```python
from build123d import *

# Parameters (mm, degrees)
SKETCH_1_W          = 10
SKETCH_1_H          = 10
EXTRUDE_1_DEPTH     = 10
SKETCH_4_R          = 3
CUT_EXTRUDE_2_DEPTH = 11
SKETCH_5_R          = 2.5
CUT_EXTRUDE_3_DEPTH = 11
FILLET_1_R          = 0.5


with BuildPart() as part:
    # 草图1 → 凸台-拉伸1 (new body)
    with BuildSketch(Plane.XY):
        with Locations((5, 5)):
            Rectangle(SKETCH_1_W, SKETCH_1_H)
    extrude(amount=EXTRUDE_1_DEPTH)

    # 草图4 → 切除-拉伸2 (cut, through all)
    with BuildSketch(Plane(origin=(10, 0, 0), x_dir=(0, 0, -1), z_dir=(1, 0, 0))):
        with Locations((-5, 5)):
            Circle(SKETCH_4_R)
    extrude(amount=-CUT_EXTRUDE_2_DEPTH, mode=Mode.SUBTRACT)

    # 草图5 → 切除-拉伸3 (cut, through all)
    with BuildSketch(Plane.XY.offset(10)):
        with Locations((5, 5)):
            Circle(SKETCH_5_R)
    extrude(amount=-CUT_EXTRUDE_3_DEPTH, mode=Mode.SUBTRACT)

    # 圆角1
    fillet_1_edges = [part.edges().sort_by_distance(p)[0] for p in [
        (10, 5, 10),
        (0, 5, 8),
        (10, 5, 8),
        (5, 10, 10),
        (2.5, 5, 0),
        (2.5, 5, 10),
        (0, 5, 10),
        (5, 10, 0),
        (10, 5, 0),
        (5, 0, 0),
        (0, 5, 0),
        (10, 10, 5),
        (10, 0, 5),
        (5, 0, 10),
    ]]
    fillet(fillet_1_edges, radius=FILLET_1_R)


solid = part.part
```
Here's how the part is built. I have some questions about the finished solid (model axes, mm). Coordinates: 2 decimals unless noted, no trailing zeros. Loops run counter-clockwise (first coordinate to the right, second up) from the corner with the lowest first, then second, coordinate; pieces in that order, holes last. Notation, with made-up numbers: (14.5, 32.5) - (60.5, 32.5) arc R20 ccw to (60.5, 71.5) - close; hole circle Ø1 at (8, 42). An arc over 180 degrees is marked (long way). Return JSON: item names as keys, results as strings. Group by question number.
Item 1: We'd pull the mould along Y, two halves only. Please class faces 1 (the face through (5, 10, 5)), 2 (the face through (2, 6, 0)), 3 (the face through (7.385, 5.751, 8.415)): +Y half, -Y half, draft (parallel to the pull), parting line (faces both ways), or undercut.
Item 2: If we section it at D-D on x = 9.25: Write out the boundary of the cut face in (y, z), and give its area (3 significant figures).
Item 3: If we section it at A-A on x = 5: Write out the boundary of the cut face in (y, z).
Item 4: If we section it at C-C on y = 5: Write out the boundary of the cut face in (x, z), and give its area (3 significant figures).
Item 5: I need wall thicknesses on line 1 (Y direction, x = 1.5, z = 7.5); line 2 (Y direction, x = 5, z = 1.65). Which ranges of each line are inside material? Lowest first, please. Write a range as from..to.
Item 6: If we section it at B-B on z = 5: Write out the boundary of the cut face in (x, y).
Calculated:
{
 "1": {"face 1": "+Y half", "face 2": "draft", "face 3": "undercut"},
 "2": {"outline": "(0, 0.5) arc R0.5 ccw to (0.5, 0) - (9.5, 0) arc R0.5 ccw to (10, 0.5) - (10, 9.5) arc R0.5 ccw to (9.5, 10) - (0.5, 10) arc R0.5 ccw to (0, 9.5) - close; hole circle Ø6 at (5, 5)", "area": "71.5 mm^2"},
 "3": {"outline": "(0, 0.5) arc R0.5 ccw to (0.5, 0) - (2, 0) arc R0.5 ccw to (2.5, 0.5) - (2.5, 3.34) arc R3 cw to (2.5, 6.66) - (2.5, 9.5) arc R0.5 ccw to (2, 10) - (0.5, 10) arc R0.5 ccw to (0, 9.5) - close; (7.5, 0.5) arc R0.5 ccw to (8, 0) - (9.5, 0) arc R0.5 ccw to (10, 0.5) - (10, 9.5) arc R0.5 ccw to (9.5, 10) - (8, 10) arc R0.5 ccw to (7.5, 9.5) - (7.5, 6.66) arc R3 cw to (7.5, 3.34) - close"},
 "4": {"outline": "(0, 0.5) arc R0.5 ccw to (0.5, 0) - (2, 0) arc R0.5 ccw to (2.5, 0.5) - (2.5, 2) - (0.5, 2) arc R0.5 ccw to (0, 1.5) - close; (0, 8.5) arc R0.5 ccw to (0.5, 8) - (2.5, 8) - (2.5, 9.5) arc R0.5 ccw to (2, 10) - (0.5, 10) arc R0.5 ccw to (0, 9.5) - close; (7.5, 0.5) arc R0.5 ccw to (8, 0) - (9.5, 0) arc R0.5 ccw to (10, 0.5) - (10, 1.5) arc R0.5 ccw to (9.5, 2) - (7.5, 2) - close; (7.5, 8) - (9.5, 8) arc R0.5 ccw to (10, 8.5) - (10, 9.5) arc R0.5 ccw to (9.5, 10) - (8, 10) arc R0.5 ccw to (7.5, 9.5) - close", "area": "19.4 mm^2"},
 "5": {"line 1": "y = 0..3.34, 6.66..10", "line 2": "y = 0..2.5, 7.5..10"},
 "6": {"outline": "(0, 0) - (9.5, 0) arc R0.5 ccw to (10, 0.5) - (10, 1.5) arc R0.5 ccw to (9.5, 2) - (0.5, 2) arc R0.5 ccw to (0, 1.5) - close; (0, 8.5) arc R0.5 ccw to (0.5, 8) - (9.5, 8) arc R0.5 ccw to (10, 8.5) - (10, 9.5) arc R0.5 ccw to (9.5, 10) - (0, 10) - close"}
}
